from build123d import *

# Parameters (mm, degrees)
REVOLVE1_ANGLE           = 180
CUT_EXTRUDE1_DEPTH       = 52
BOSS_EXTRUDE1_REACH      = 25.5
BOSS_EXTRUDE1_END_RADIUS = 17.5
SKETCH7_R                = 3


with BuildPart() as part:
    # Sketch3 → Revolve1 (revolve)
    with BuildSketch(Plane.XY):
        Polygon((0, 0), (25.5, 0), (25.5, 7.5), (19, 7.5), (19, 14.5), (17.5, 14.5), (17.5, 36.5), (19, 36.5), (19, 43.5), (25.5, 43.5), (25.5, 51), (0, 51), align=None)
    revolve(axis=Axis((0, 0, 0), (0, 1, 0)), revolution_arc=REVOLVE1_ANGLE)

    # Sketch4 → Cut-Extrude1 (cut, through all)
    with BuildSketch(Plane(origin=(0, 51, 0), x_dir=(1, 0, 0), z_dir=(0, 1, 0))):
        with BuildLine():
            Line((-12.5, 0), (12.5, 0))
            ThreePointArc((12.5, 0), (0, 12.5), (-12.5, 0))
        make_face()
    extrude(amount=-CUT_EXTRUDE1_DEPTH, mode=Mode.SUBTRACT)

    # Boss-Extrude1: up to this cylinder (the profile starts outside it)
    boss_extrude1_end = Plane(origin=(0, 25.5, 0), z_dir=(0, -1, 0)) * Cylinder(BOSS_EXTRUDE1_END_RADIUS, 87, mode=Mode.PRIVATE)
    # Sketch7 → Boss-Extrude1 (add, up to the surface)
    with BuildSketch(Plane(origin=(0, 0, -23.5), x_dir=(-1, 0, 0), z_dir=(0, 0, -1)), mode=Mode.PRIVATE) as boss_extrude1_sk1:
        with Locations((0, 25.5)):
            Circle(SKETCH7_R)
    boss_extrude1_tool1 = extrude(boss_extrude1_sk1.sketch, amount=-BOSS_EXTRUDE1_REACH, mode=Mode.PRIVATE) - boss_extrude1_end
    add(boss_extrude1_tool1.solids().sort_by_distance((0, 25.5, -23.5))[0])


solid = part.part
For this review, take the finished solid that the model builds, in its own axes (mm). A direction names the side the tool comes from. Coordinates: 2 decimals unless noted, no trailing zeros. Write each loop counter-clockwise with the first axis right and the second up, starting at its lowest first coordinate (ties: lowest second). Pieces come first, ordered by that corner, then holes. Notation, with made-up numbers: (6.5, -21.75) -> (33.5, -21.75) arc R5 cw to (33.5, -17.75) -> close; hole circle Ø9 at (42, 72). An arc over 180 degrees is marked (long way). Write each question's results on one line, items separated by ' | '. Start each with the question number.
1) Consider section A-A (z = -22). Write out the cut boundary in (x, y), plus the area to 3 significant figures.
2) Consider section B-B (x = 0). Write out the cut boundary in (y, z), plus the area to 3 significant figures.
3) Consider section D-D (x = 15.5). Write out the cut boundary in (y, z), plus the area to 3 significant figures.
4) Wall thickness on L1, parallel to Y at x = -21, z = -10.75; L2, parallel to Y at x = 16.5, z = -7.75; L3, parallel to Z at x = -0.5, y = 12.5: over which ranges is each line inside the solid? List them lowest first. Write a range as [from, to].
5) Consider section C-C (y = 25.5). Write out the cut boundary in (x, z).
6) Insertion check: pin 1 (7.5 mm diameter, centred on x = 6, z = -16.5, fed in from -Y); pin 2 (9.5 mm diameter, centred on x = 4, z = -5.5, fed in from -Y); pin 3 (5 mm diameter, centred on y = 44, z = -20.5, fed in from +X); pin 4 (5 mm diameter, centred on y = 8, z = -3, fed in from -X). Each pin has a flat end and moves straight along its axis. Give the tip position at first contact, or say it passes through.
7) For faces 1 (the face through (0.65, 22.57, -20.41)), 2 (the face through (0.561, 3.802, -25.494)), 3 (the face through (0, 26, -23.5)), list the 3-axis set-ups (+Z, -Z, +X, -X, +Y, -Y) from which the entire face can be reached by the end or side of a thin tool; tool diameter is ignored.
8) The part is to be moulded in two halves that separate along Y. For faces 4 (the face through (6.346, 25.654, -16.309)), 5 (the face through (17, 26, 0)), 6 (the face through (0, 51, -13)), say which applies: +Y half, -Y half, draft (parallel to the pull), parting line (faces both ways), or undercut.
Geometry says:
1) outline: (-12.89, 0) -> (12.89, 0) -> (12.89, 7.5) -> (-12.89, 7.5) -> close; (-12.89, 43.5) -> (12.89, 43.5) -> (12.89, 51) -> (-12.89, 51) -> close; circle Ø6 at (0, 25.5) | area: 415 mm^2
2) outline: (0, -25.5) -> (7.5, -25.5) -> (7.5, -19) -> (14.5, -19) -> (14.5, -17.5) -> (22.5, -17.5) -> (22.5, -23.5) -> (28.5, -23.5) -> (28.5, -17.5) -> (36.5, -17.5) -> (36.5, -19) -> (43.5, -19) -> (43.5, -25.5) -> (51, -25.5) -> (51, -12.5) -> (0, -12.5) -> close | area: 432 mm^2
3) outline: (0, -20.25) -> (7.5, -20.25) -> (7.5, -10.99) -> (14.5, -10.99) -> (14.5, -8.12) -> (36.5, -8.12) -> (36.5, -10.99) -> (43.5, -10.99) -> (43.5, -20.25) -> (51, -20.25) -> (51, 0) -> (0, 0) -> close | area: 636 mm^2
4) L1: [0, 7.5], [43.5, 51] | L2: [0, 14.5], [36.5, 51] | L3: [-18.99, -12.49]
5) outline: (-17.5, 0) arc R17.5 ccw to (-3, -17.24) -> (-3, -23.5) -> (3, -23.5) -> (3, -17.24) arc R17.5 ccw to (17.5, 0) -> (12.5, 0) arc R12.5 cw to (-12.5, 0) -> close
6) pin 1: y = 0 | pin 2: through | pin 3: x = 18.06 | pin 4: x = -25.49
7) face 1: -Z | face 2: -Z, +Y, -Y | face 3: -Z, +X, -X
8) face 4: undercut | face 5: draft | face 6: +Y half
